Geometry check sheet. Reference: the model listing, model coordinates, mm. Face numbers are marked on the shaded views. A direction names the side the tool comes from. Round coordinates to 2 decimals unless told otherwise and drop trailing zeros. Order: outer loops, then holes, each group sorted by start corner. A loop starts at its lowest first (then second) coordinate and runs counter-clockwise, first axis right, second up.
(1) Cross-section at D-D on x = -91. Enter the section's corners in (y, z).
(2) Cross-section at C-C on y = 39. Count the separate pieces of the cut face and the enclosed holes in it, and give its area (3 significant figures).
(3) Cross-section at A-A on y = -26. Enter the section's corners in (x, z), and give its area (3 significant figures).
(4) Set-up check for the marked faces 1, 2, 3 and 4: record each of +Z, -Z, +X, -X, +Y, -Y from which the full face is reachable in a straight line by a thin tool's end or side.
(5) Gauge pin test, flat ends, axial feed: P1, Ø1.5, axis at x = -32.5, z = 23.5, coming from the +Y side; P2, Ø10, axis at x = 20.5, z = 24, coming from the +Y side; P3, Ø1.5, axis at x = -59.5, z = 26, coming from the -Y side. Record the tip position at first contact, or that the pin passes through.
(6) Cross-section at B-B on z = 32.5. Enter the section's corners in (x, y), and give its area (3 significant figures).
(7) Thickness scan on L1, parallel to X at y = 40.5, z = 34.5; L2, parallel to Y at x = 2.5, z = 20; L3, parallel to X at y = 28, z = 27. Record the ranges inside material, lowest first.
(8) Draft check along X on the marked faces 5, 6 and 7. Enter one of: pulls with the +X half, pulls with the -X half, needs draft (parallel to the pull), parting line crosses it, or undercut.
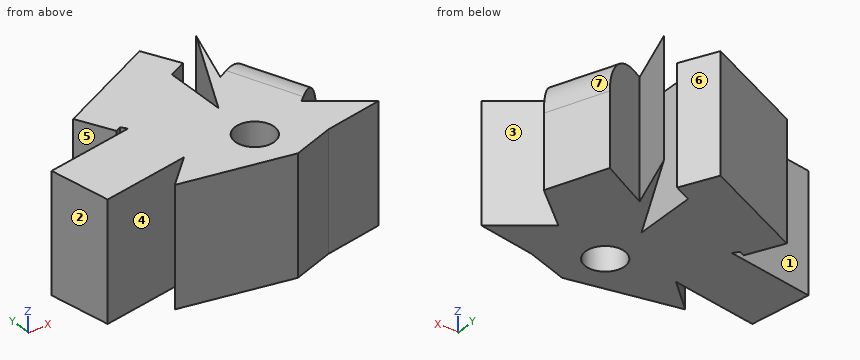
from build123d import *

# Parameters (mm, degrees)
F1_DEPTH = 77.216
F2_R     = 29.4340917525
F4_D     = 25.4
F5_DEPTH = 25.654
F6_DEPTH = 57.912


with BuildPart() as f1:
    # F0 (on Top) → F1 (new body)
    with BuildSketch(Plane.XY):
        Polygon((32.8288413584, 64.337939024), (0, 0), (0, 69.9468851089), (-67.8022876382, 36.6231352091), (-50.315566361, 11.8777733296), (-43.3868691325, -28.3746812493), (-63.5130926967, -47.5110933185), (7.0936689153, -60.7086196542), (34.1485999525, -51.1404126883), (71.7615485191, -44.2117117345), (39.4276119769, -20.1262254268), (66.1525949836, 3.2993813511), (51.3053834438, 41.5722057223), (18.9714413136, 24.0854844451), align=None)
    extrude(amount=F1_DEPTH)

    # F2
    f2_edges = [f1.edges().sort_by_distance(p)[0] for p in [
        (58.728989, 22.435794, 77.216),
    ]]
    fillet(f2_edges, radius=F2_R)

    # F4 (through all)
    with Locations(Plane.XY.offset(77.216)):
        with Locations((0, -32.1689685807)):
            Hole(F4_D / 2)

    # F5 (add): a face of the model
    f5_faces = [f1.faces().sort_by_distance(p)[0] for p in [
        (-33.9011438191, 53.285010159, 38.608),
    ]]
    extrude(f5_faces, amount=-F5_DEPTH)

    # F6 (add): a face of the model
    f6_faces = [f1.faces().sort_by_distance(p)[0] for p in [
        (-46.8512177467, -8.2484539598, 38.608),
    ]]
    extrude(f6_faces, amount=F6_DEPTH)


solid = f1.part
Found:
1. outline: (-36.57, 0) - (4.87, 0) - (4.87, 77.22) - (-36.57, 77.22) - close
2. separate pieces: 3
2. enclosed holes: 0
2. area: 5,530 mm2
3. outline: (-102.56, 0) - (-11.1, 0) - (-11.1, 77.22) - (-102.56, 77.22) - close; (11.1, 0) - (47.31, 0) - (47.31, 77.22) - (11.1, 77.22) - close
3. area: 9,860 mm2
4. face 1: +Z, -Z, -X
4. face 2: +Z, -Z, -X, -Y
4. face 3: +Z, -Z, +X
4. face 4: +Z, -Z
5. P1: stops at y = 54.34
5. P2: stops at y = 49.97
5. P3: stops at y = -48.4
6. outline: (-107.39, 2.05) - (-100.46, -38.2) - (-43.39, -28.37) - (-63.51, -47.51) - (7.09, -60.71) - (34.15, -51.14) - (71.76, -44.21) - (39.43, -20.13) - (66.15, 3.3) - (51.31, 41.57) - (18.97, 24.09) - (32.83, 64.34) - (0, 0) - (0, 41.36) - (11.32, 46.92) - (0, 69.95) - (-67.8, 36.62) - (-56.49, 13.6) - (-52.81, 15.41) - (-50.32, 11.88) - close; hole circle Ø25.4 at (0, -32.17)
6. area: 12,700 mm2
7. L1: x = -59.91 to 0, 20.67 to 24.62, 49.32 to 51.72
7. L2: y = -59.85 to -44.62, -19.72 to 4.9, 42.59 to 64.86
7. L3: x = -63.56 to 0, 14.29 to 20.32, 26.21 to 56.57
8. face 5: pulls with the -X half
8. face 6: undercut
8. face 7: pulls with the +X half
